Can you work these out from the model? Positions are in its coordinate system, mm. Face numbers are marked on the shaded views. A direction names the side the tool comes from. Round coordinates to 2 decimals unless told otherwise and drop trailing zeros. Write each loop counter-clockwise with the first axis right and the second up, starting at its lowest first coordinate (ties: lowest second). Pieces come first, ordered by that corner, then holes. Notation, with made-up numbers: (13, -5.75) -> (69, -5.75) arc R7 ccw to (69, 2.25) -> close; hole circle Ø5 at (32, -12). An arc over 180 degrees is marked (long way). Use CSV: the item, a comma, the result in double quotes.
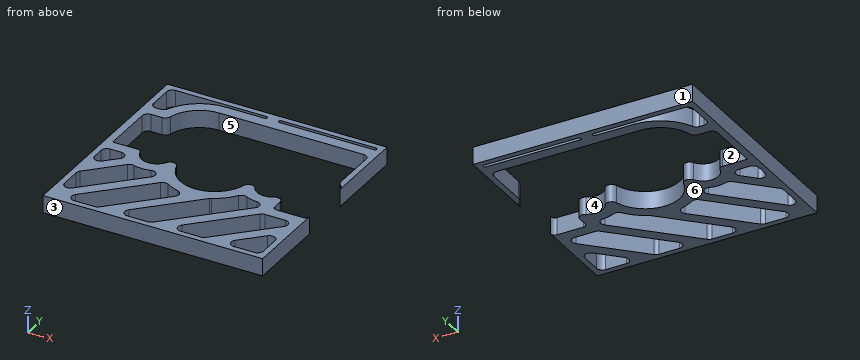
```python
from build123d import *

# Parameters (mm, degrees)
PAD_DEPTH = 1.5


with BuildPart() as part:
    # Sketch → Pad (new body)
    with BuildSketch(Plane.XY):
        with BuildLine():
            ThreePointArc((-2.8995, -0.77), (0, -3), (2.8995, -0.77))
            ThreePointArc((3.819845, -0.65554), (3.321042, -0.402156), (2.8995, -0.77))
            ThreePointArc((3.819845, -0.65554), (4.670792, -1.309245), (5.72973, -1.135779))
            ThreePointArc((6.5, -1.556438), (6.239651, -1.117613), (5.72973, -1.135779))
            Line((6.5, -2.35), (6.5, -1.556438))
            ThreePointArc((6.5, -2.35), (6.602513, -2.597487), (6.85, -2.7))
            Line((6.85, -2.7), (9.15, -2.7))
            ThreePointArc((9.15, -2.7), (9.397487, -2.597487), (9.5, -2.35))
            Line((9.5, -2.35), (9.5, -9.5))
            Line((-9.5, -9.5), (9.5, -9.5))
            Line((-9.5, 9.5), (-9.5, -9.5))
            Line((9.5, 9.5), (-9.5, 9.5))
            Line((9.5, 2.35), (9.5, 9.5))
            ThreePointArc((9.5, 2.35), (9.434288, 2.639872), (9.25, 2.873071))
            ThreePointArc((9, 3.396143), (9.065712, 3.106271), (9.25, 2.873071))
            Line((9, 3.396143), (9, 7.2))
            ThreePointArc((9, 7.2), (8.853553, 7.553553), (8.5, 7.7))
            Line((8.5, 7.7), (-4, 7.7))
            ThreePointArc((-4, 7.7), (-5.863177, 7.051291), (-6.920581, 5.385714))
            ThreePointArc((-7.407345, 5), (-7.096816, 5.108118), (-6.920581, 5.385714))
            Line((-8.35, 5), (-7.407345, 5))
            ThreePointArc((-8.35, 5), (-8.703553, 4.853553), (-8.85, 4.5))
            Line((-8.85, 0), (-8.85, 4.5))
            Line((-8.85, 0), (-6.722884, 0))
            ThreePointArc((-6.310819, -0.322882), (-6.461135, -0.090335), (-6.722884, 0))
            ThreePointArc((-6.310819, -0.322882), (-5.1787, -1.33812), (-3.819845, -0.65554))
            ThreePointArc((-2.8995, -0.77), (-3.321042, -0.402156), (-3.819845, -0.65554))
        make_face()
        with BuildLine():
            Line((-8.146447, -7.43934), (-3.773762, -3.066655))
            ThreePointArc((-3.773762, -3.066655), (-3.70061, -2.452483), (-4.280418, -2.237119))
            ThreePointArc((-5.735884, -2.23181), (-5.008573, -2.349984), (-4.280418, -2.237119))
            ThreePointArc((-5.735884, -2.23181), (-6.008123, -2.220226), (-6.246009, -2.353109))
            Line((-8.853553, -4.960654), (-6.246009, -2.353109))
            ThreePointArc((-8.853553, -4.960654), (-8.96194, -5.122866), (-9, -5.314207))
            Line((-9, -5.314207), (-9, -7.085786))
            ThreePointArc((-9, -7.085786), (-8.691342, -7.547726), (-8.146447, -7.43934))
        make_face(mode=Mode.SUBTRACT)
        with BuildLine():
            Line((-7.43934, -8.146447), (-2.748865, -3.455972))
            ThreePointArc((-2.129166, -3.386245), (-2.451218, -3.312661), (-2.748865, -3.455972))
            ThreePointArc((-2.129166, -3.386245), (-1.598864, -3.666556), (-1.032607, -3.864417))
            ThreePointArc((-0.80813, -4.701023), (-0.678765, -4.217893), (-1.032607, -3.864417))
            Line((-4.96066, -8.853553), (-0.80813, -4.701023))
            ThreePointArc((-5.314214, -9), (-5.122872, -8.96194), (-4.96066, -8.853553))
            Line((-5.314214, -9), (-7.085786, -9))
            ThreePointArc((-7.43934, -8.146447), (-7.547726, -8.691342), (-7.085786, -9))
        make_face(mode=Mode.SUBTRACT)
        with BuildLine():
            Line((-7.51422, -1), (-8.5, -1))
            ThreePointArc((-8.5, -1), (-8.853553, -1.146447), (-9, -1.5))
            Line((-9, -1.5), (-9, -2.48578))
            ThreePointArc((-9, -2.48578), (-8.691342, -2.94772), (-8.146447, -2.839334))
            Line((-8.146447, -2.839334), (-7.160666, -1.853553))
            ThreePointArc((-7.160666, -1.853553), (-7.05228, -1.308658), (-7.51422, -1))
        make_face(mode=Mode.SUBTRACT)
        with BuildLine():
            ThreePointArc((1.748237, -3.597731), (2.611317, -3.03002), (3.300222, -2.260206))
            ThreePointArc((3.938583, -2.096639), (3.588644, -2.058379), (3.300222, -2.260206))
            ThreePointArc((3.938583, -2.096639), (4.428947, -2.279561), (4.947635, -2.349417))
            ThreePointArc((5.290047, -3.202846), (5.400537, -2.66311), (4.947635, -2.349417))
            Line((5.290047, -3.202846), (-0.36066, -8.853553))
            ThreePointArc((-0.714214, -9), (-0.522872, -8.96194), (-0.36066, -8.853553))
            Line((-0.714214, -9), (-2.485786, -9))
            ThreePointArc((-2.83934, -8.146447), (-2.947726, -8.691342), (-2.485786, -9))
            Line((-2.83934, -8.146447), (1.613213, -3.693894))
            ThreePointArc((1.748237, -3.597731), (1.676712, -3.640178), (1.613213, -3.693894))
        make_face(mode=Mode.SUBTRACT)
        with BuildLine():
            ThreePointArc((8.5, -9), (8.853553, -8.853553), (9, -8.5))
            Line((9, -6.714214), (9, -8.5))
            ThreePointArc((9, -6.714214), (8.691342, -6.252274), (8.146447, -6.36066))
            Line((6.36066, -8.146447), (8.146447, -6.36066))
            ThreePointArc((6.36066, -8.146447), (6.252274, -8.691342), (6.714214, -9))
            Line((6.714214, -9), (8.5, -9))
        make_face(mode=Mode.SUBTRACT)
        with BuildLine():
            Line((8.185786, -3.7), (6.414214, -3.7))
            ThreePointArc((6.414214, -3.7), (6.222872, -3.73806), (6.06066, -3.846447))
            Line((6.06066, -3.846447), (1.76066, -8.146447))
            ThreePointArc((1.76066, -8.146447), (1.652274, -8.691342), (2.114214, -9))
            Line((3.885786, -9), (2.114214, -9))
            ThreePointArc((3.885786, -9), (4.077128, -8.96194), (4.23934, -8.853553))
            Line((4.23934, -8.853553), (8.53934, -4.553553))
            ThreePointArc((8.53934, -4.553553), (8.647726, -4.008658), (8.185786, -3.7))
        make_face(mode=Mode.SUBTRACT)
        with BuildLine():
            Line((-9, 8.5), (-9, 6.5))
            ThreePointArc((-9, 6.5), (-8.853553, 6.146447), (-8.5, 6))
            Line((-8.5, 6), (-8.124318, 6))
            ThreePointArc((-8.124318, 6), (-7.850457, 6.08167), (-7.666061, 6.3))
            ThreePointArc((-4, 8.7), (-6.19089, 8.04664), (-7.666061, 6.3))
            Line((-4, 8.7), (-0.65, 8.7))
            ThreePointArc((-0.65, 8.7), (-0.5, 8.85), (-0.65, 9))
            Line((-8.5, 9), (-0.65, 9))
            ThreePointArc((-8.5, 9), (-8.853553, 8.853553), (-9, 8.5))
        make_face(mode=Mode.SUBTRACT)
        with BuildLine():
            ThreePointArc((8.85, 8.7), (9, 8.85), (8.85, 9))
            Line((0.65, 9), (8.85, 9))
            ThreePointArc((0.65, 9), (0.5, 8.85), (0.65, 8.7))
            Line((0.65, 8.7), (8.85, 8.7))
        make_face(mode=Mode.SUBTRACT)
    extrude(amount=PAD_DEPTH)


solid = part.part
```
Q1. Suppose I cut it at D-D (z = 1). Count the separate pieces of the cut face and the enclosed holes in it, and give its area (3 significant figures).
Resolved:
separate pieces,"1"
enclosed holes,"8"
area,"114 mm^2"
Q2. Will this pin go through, and if not, where does the flat tip stop? P1, Ø1.5, axis at x = -2, y = 1, coming from the -Z side.
Resolved:
P1,"passes through"
Q3. Suppose I cut it at C-C (y = 1). Write out the boundary of the cut face in (x, z).
Resolved:
outline,"(-9.5, 0) -> (-8.85, 0) -> (-8.85, 1.5) -> (-9.5, 1.5) -> close"
Q4. Suppose I cut it at A-A (y = 4). Write out the boundary of the cut face in (x, z).
Resolved:
outline,"(-9.5, 0) -> (-8.85, 0) -> (-8.85, 1.5) -> (-9.5, 1.5) -> close; (9, 0) -> (9.5, 0) -> (9.5, 1.5) -> (9, 1.5) -> close"
Q5. If we mould it in two halves opening along Y, with no side actions, what happens to the marked faces 1, 2, 3 and 4? For each: released by +Y, released by -Y, zero draft, split by the parting line, or undercut.
Resolved:
face 1,"released by +Y"
face 2,"undercut"
face 3,"released by -Y"
face 4,"undercut"
Q6. Please list where these lines run through material, in increasing order: probe 1 along X at (y, z) = (-6, 0.25); probe 2 along Y at (x, z) = (1.5, 0.1); probe 3 along Y at (x, z) = (6.75, 0.95).
Resolved:
probe 1,"x = -9.5 to -9, -6.71 to -5.29, -2.11 to -0.69, 2.49 to 3.91, 7.09 to 9.5"
probe 2,"y = -9.5 to -6.99, -3.81 to -2.6, 7.7 to 8.7, 9 to 9.5"
probe 3,"y = -9.5 to -9, -7.76 to -6.34, -3.7 to -2.69, 7.7 to 8.7, 9 to 9.5"
Q7. Suppose I cut it at B-B (x = 2.5). Write out the boundary of the cut face in (y, z), and give its area (3 significant figures).
Resolved:
outline,"(-9.5, 0) -> (-9, 0) -> (-9, 1.5) -> (-9.5, 1.5) -> close; (-7.41, 0) -> (-5.99, 0) -> (-5.99, 1.5) -> (-7.41, 1.5) -> close; (-3.12, 0) -> (-1.66, 0) -> (-1.66, 1.5) -> (-3.12, 1.5) -> close; (7.7, 0) -> (8.7, 0) -> (8.7, 1.5) -> (7.7, 1.5) -> close; (9, 0) -> (9.5, 0) -> (9.5, 1.5) -> (9, 1.5) -> close"
area,"7.32 mm^2"
Q8. On a 3-axis mill with a long thin cutter (end or side, diameter ignored), from which of +Z, -Z, +X, -X, +Y, -Y can I reach the whole of each face in a straight line? I mean the marked faces 5 and 6. Say none if no direction works.
Resolved:
face 5,"+Z, -Z"
face 6,"-Z, +X, -X, +Y, -Y"
